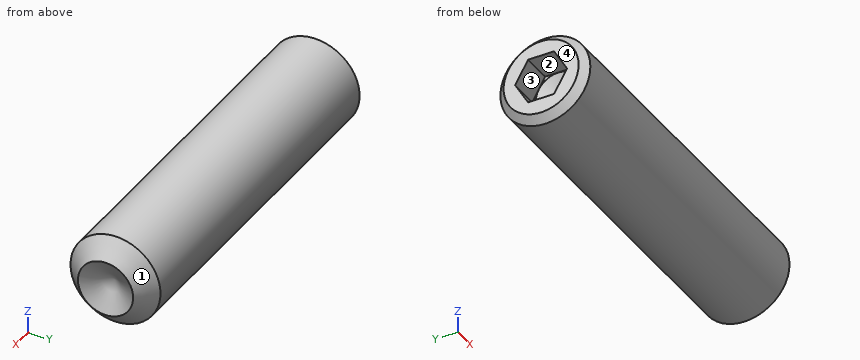
from build123d import *

# Parameters (mm, degrees)
SKETCH1_W          = 25
SKETCH1_H          = 3
CUT_EXTRUDE1_DEPTH = 2
CHAMFER1_SIZE      = 0.5
CHAMFER2_SIZE      = 1.25


with BuildPart() as part:
    # Sketch1 → Revolve1 (revolve)
    with BuildSketch(Plane.XY, mode=Mode.PRIVATE) as revolve1_sk:
        with Locations((12.5, 1.5)):
            Rectangle(SKETCH1_W, SKETCH1_H)
    revolve(revolve1_sk.sketch.rotate(Axis((25, 0, 0), (-1, 0, 0)), 180), axis=Axis((25, 0, 0), (-1, 0, 0)))

    # Sketch2 → Cut-Revolve1 (revolve, cut)
    with BuildSketch(Plane.XY, mode=Mode.PRIVATE) as cut_revolve1_sk:
        Polygon((2, 1.495), (2.863138652, 0), (0, 0), (0, 1.495), align=None)
    revolve(cut_revolve1_sk.sketch.rotate(Axis((-1.178327448, 0, 0), (1, 0, 0)), 270), axis=Axis((-1.178327448, 0, 0), (1, 0, 0)), mode=Mode.SUBTRACT)

    # Sketch3 → Cut-Extrude1 (cut)
    with BuildSketch(Plane.ZY):
        Polygon((0, 1.732050808), (-1.5, 0.866025404), (-1.5, -0.866025404), (0, -1.732050808), (1.5, -0.866025404), (1.5, 0.866025404), align=None)
    extrude(amount=-CUT_EXTRUDE1_DEPTH, mode=Mode.SUBTRACT)

    # Sketch4 → Cut-Revolve2 (revolve, cut)
    with BuildSketch(Plane.XY, mode=Mode.PRIVATE) as cut_revolve2_sk:
        Polygon((25, 1.995), (25, 0), (23.848186213, 0), align=None)
    revolve(cut_revolve2_sk.sketch.rotate(Axis((-1.256465595, 0, 0), (1, 0, 0)), 90), axis=Axis((-1.256465595, 0, 0), (1, 0, 0)), mode=Mode.SUBTRACT)

    # Chamfer1
    chamfer1_edges = [part.edges().sort_by_distance(p)[0] for p in [
        (0, 3, 0),
    ]]
    chamfer(chamfer1_edges, length=CHAMFER1_SIZE)

    # Chamfer2
    # the kernel refuses this chamfer: 1.25 mm, written as the material it takes off along each edge
    with BuildSketch(Plane(origin=(25, 0, 0), x_dir=(0, -1, 0), z_dir=(0, 0, -1))) as chamfer2_piece_1:
        Polygon((3, CHAMFER2_SIZE), (3 - CHAMFER2_SIZE, 0), (3, 0), align=None)
    revolve(axis=Axis((25, 0, 0), (-1, 0, 0)), mode=Mode.SUBTRACT)


solid = part.part
Can you work these out from the model? Positions are in its coordinate system, mm. Face numbers are marked on the shaded views. Round coordinates to 2 decimals unless told otherwise and drop trailing zeros. Write each loop counter-clockwise with the first axis right and the second up, starting at its lowest first coordinate (ties: lowest second). Pieces come first, ordered by that corner, then holes. Notation, with made-up numbers: (42, 4) - (56, 4) arc R22 ccw to (56, 26) - close; hole circle Ø8 at (54.25, -35.75). An arc over 180 degrees is marked (long way). Write each question's results on one line, items separated by ' | '. Start each with the question number.
1) Please list where these lines run through material, in increasing order: line 1 (Y direction, x = 20, z = 2.45); line 2 (Z direction, x = 2.5, y = 0.1); line 3 (Z direction, x = 10, y = -1.1).
2) Suppose I cut it at A-A (x = 20). List the corners of the cut face in (y, z) for me.
3) For pin 1 Ø0.5 at (x, y) = (0.5, -0.5) entering from -Z; pin 2 Ø1.5 at (y, z) = (0, 0.5) entering from -X; pin 3 Ø1 at (x, z) = (8, -1) entering from -Y, each with a flat end and sliding along its axis, tell me the tip position at first contact or that it passes through.
4) We'd pull the mould along Y, two halves only. Please class the marked faces 1, 2, 3 and 4: released by +Y, released by -Y, zero draft, split by the parting line, or undercut.
Here are the results:
1) line 1: y = -1.73 to 1.73 | line 2: z = -3 to -0.62, 0.62 to 3 | line 3: z = -2.79 to 2.79
2) outline: circle Ø6 at (0, 0)
3) pin 1: stops at z = -2.99 | pin 2: stops at x = 2.14 | pin 3: stops at y = -2.96
4) face 1: split by the parting line | face 2: undercut | face 3: undercut | face 4: zero draft
